```python
from build123d import *

# Parameters (mm, degrees)
F0_R     = 6
F0_R_2   = 21
F1_DEPTH = 10


with BuildPart() as f1:
    # F0 (on Top) → F1 (new body)
    with BuildSketch(Plane.XY):
        with BuildLine():
            Line((-41.271994, -13.625788), (-12.858001, -27.10483))
            ThreePointArc((-12.858001, -27.10483), (-0.858643, -29.98771), (11.286012, -27.796149))
            Line((11.286012, -27.796149), (39.195127, -14.40142))
            ThreePointArc((39.195127, -14.40142), (49.952353, -1.194627), (41.428532, 13.552637))
            Line((41.428532, 13.552637), (12.924047, 27.0734))
            Line((12.924047, 27.0734), (12.790003, 27.136983))
            ThreePointArc((12.790003, 27.136983), (0.947593, 29.985031), (-11.051015, 27.890412))
            Line((-11.051015, 27.890412), (-42.937387, 12.727839))
            ThreePointArc((-42.937387, 12.727839), (-49.970138, -0.946024), (-41.271994, -13.625788))
        make_face()
        with Locations((-35, 0)):
            Circle(F0_R, mode=Mode.SUBTRACT)
        Circle(F0_R_2, mode=Mode.SUBTRACT)
        with Locations((35, 0)):
            Circle(F0_R, mode=Mode.SUBTRACT)
    extrude(amount=F1_DEPTH)


solid = f1.part
```
The listing builds one solid part. Answer for the finished solid, in the listing's coordinates (mm). Give positions to 0.01 mm unless a question says otherwise; leave off trailing zeros. Order: outer loops, then holes, each group sorted by start corner. A loop starts at its lowest first (then second) coordinate and runs counter-clockwise, first axis right, second up.
Item 1: The part is cut by section B-B, the plane x = 0. Give the vertices of the cut face in (y, z), and give its area (3 significant figures).
From the geometry:
outline: (-30, 0) - (-21, 0) - (-21, 10) - (-30, 10) - close; (21, 0) - (30, 0) - (30, 10) - (21, 10) - close
area: 180 mm2
Item 2: The part is cut by section C-C, the plane y = 0. Give the vertices of the cut face in (x, z).
From the geometry:
outline: (-50, 0) - (-41, 0) - (-41, 10) - (-50, 10) - close; (-29, 0) - (-21, 0) - (-21, 10) - (-29, 10) - close; (21, 0) - (29, 0) - (29, 10) - (21, 10) - close; (41, 0) - (50, 0) - (50, 10) - (41, 10) - close
Item 3: For a pull along Y with two mould halves and no side action, classify faces 1 (the face through (20.03, 6.31, 4.93)), 2 (the face through (30.24, -3.65, 4.93)), 3 (the face through (49.93, -1.45, 4.93)), 4 (the face through (22, 0, 0)) as pulls with the +Y half, pulls with the -Y half, needs draft (parallel to the pull), parting line crosses it, or undercut.
From the geometry:
face 1: undercut
face 2: undercut
face 3: parting line crosses it
face 4: needs draft
Item 4: Find the intervals of material crossed by probe 1 along Y at (x, z) = (0, 2.75); probe 2 along X at (y, z) = (5.5, 5.5); probe 3 along X at (y, z) = (4, 2), in increasing order.
From the geometry:
probe 1: y = -30 to -21, 21 to 30
probe 2: x = -48.96 to -37.4, -32.6 to -20.27, 20.27 to 32.6, 37.4 to 48.96
probe 3: x = -49.46 to -39.47, -30.53 to -20.62, 20.62 to 30.53, 39.47 to 49.46
Item 5: The part is cut by section A-A, the plane z = 7.75. Give the vertices of the cut face in (x, y).
From the geometry:
outline: (-42.94, 12.73) arc R15 ccw to (-41.27, -13.63) - (-12.86, -27.1) arc R30 ccw to (11.29, -27.8) - (39.2, -14.4) arc R15 ccw to (41.43, 13.55) - (12.92, 27.07) - (12.79, 27.14) arc R30 ccw to (-11.05, 27.89) - close; hole circle Ø12 at (-35, 0); hole circle Ø42 at (0, 0); hole circle Ø12 at (35, 0)
Item 6: Given pin 1 Ø2 at (y, z) = (10, 5.5) entering from -X; pin 2 Ø5 at (y, z) = (-12, 3.5) entering from -X, each flat-ended and moving along its own axis, determine where each tip first touches the part or whether it passes through.
From the geometry:
pin 1: stops at x = -47
pin 2: stops at x = -46.61
Item 7: The part is cut by section D-D, the plane y = -7.5. Give the vertices of the cut face in (x, z).
From the geometry:
outline: (-47.99, 0) - (-19.62, 0) - (-19.62, 10) - (-47.99, 10) - close; (19.62, 0) - (47.99, 0) - (47.99, 10) - (19.62, 10) - close
